For this review, take the finished solid that the model builds, in its own axes (mm). A direction names the side the tool comes from. Give positions to 0.01 mm unless a question says otherwise; leave off trailing zeros. Loops run counter-clockwise (first coordinate to the right, second up) from the corner with the lowest first, then second, coordinate; pieces in that order, holes last. Notation, with made-up numbers: (-10, 34.5) -> (17, 34.5) arc R30 cw to (17, 62.5) -> close; hole circle Ø6 at (-5, 62.5). An arc over 180 degrees is marked (long way). One line per question, with ' | ' between items. Start each with the question number.
(1) Insertion check: P1, Ø4, axis at y = 8, z = -6, coming from the -X side; P2, Ø6, axis at x = -14.5, y = 10.5, coming from the +Z side; P3, Ø6, axis at x = 6.5, y = 6.5, coming from the +Z side. Each pin has a flat end and moves straight along its axis. Give the tip position at first contact, or say it passes through.
(2) Consider section A-A (z = -16). Write out the cut boundary in (x, y), and give its area (3 significant figures).
(3) Consider section B-B (x = -5.5). Write out the cut boundary in (y, z), and give its area (3 significant figures).
(4) Consider section D-D (x = 11). Write out the cut boundary in (y, z).
(5) Wall thickness on probe 1 along Z at (x, y) = (8, 13); probe 2 along Y at (x, z) = (-15, 7); probe 3 along X at (y, z) = (16, -12.5): over which ranges is each line inside the solid? List them lowest first.
(6) Consider section C-C (y = 3). Write out the cut boundary in (x, z).
(7) Tool access review of faces 1 (the flat face through (11, 14, -11)), 2 (the flat face through (-15, 14, 0)), 3 (the cylindrical face through (3.878, 14.465, -9.218)): name each direction out of +Z, -Z, +X, -X, +Y, -Y from which nothing blocks a thin tool from reaching the whole face with its end or side.
(8) Draft analysis for pull direction Z (two halves, no side actions). For faces 4 (the flat face through (0, 0, 0)), 5 (the cylindrical face through (-9.218, 14.465, -3.878)), 6 (the flat face through (-11, 14, -11)), state which applies: +Z half, -Z half, draft (parallel to the pull), parting line (faces both ways), or undercut.
from build123d import *

# Parameters (mm, degrees)
SKETCH1_R                      = 20
EXTRUDE_MECHANISM_PART_1_DEPTH = 17
CUT_START                      = -5
CUT_MECHANISM_PART_1_DEPTH     = 5


with BuildPart() as part:
    # Sketch1 → Extrude (Mechanism Part 1) (new body)
    with BuildSketch(Plane(origin=(0, 0, 0), x_dir=(1, 0, 0), z_dir=(0, 1, 0))):
        with Locations(Location((0, 0, 0), (0, 0, 270))):
            Circle(SKETCH1_R)
    extrude(amount=EXTRUDE_MECHANISM_PART_1_DEPTH)

    # Sketch2 → Cut (Mechanism Part 1) (cut)
    with BuildSketch(Plane(origin=(0, 17, 0), x_dir=(1, 0, 0), z_dir=(0, 1, 0)).offset(CUT_START)):
        with BuildLine():
            Line((0, 10), (0, 20))
            ThreePointArc((0, 20), (-7.653668647, 18.47759065), (-14.142135624, 14.142135624))
            Line((-14.142135624, 14.142135624), (-7.071067812, 7.071067812))
            ThreePointArc((-7.071067812, 7.071067812), (-3.826834324, 9.238795325), (0, 10))
        make_face()
        with BuildLine():
            ThreePointArc((20, 0), (18.47759065, 7.653668647), (14.142135624, 14.142135624))
            Line((14.142135624, 14.142135624), (7.071067812, 7.071067812))
            ThreePointArc((7.071067812, 7.071067812), (9.238795325, 3.826834324), (10, 0))
            Line((10, 0), (20, 0))
        make_face()
        with BuildLine():
            ThreePointArc((7.071067812, -7.071067812), (3.826834324, -9.238795325), (0, -10))
            Line((0, -10), (0, -20))
            ThreePointArc((0, -20), (7.653668647, -18.47759065), (14.142135624, -14.142135624))
            Line((14.142135624, -14.142135624), (7.071067812, -7.071067812))
        make_face()
        with BuildLine():
            Line((-10, 0), (-20, 0))
            ThreePointArc((-20, 0), (-18.47759065, -7.653668647), (-14.142135624, -14.142135624))
            Line((-14.142135624, -14.142135624), (-7.071067812, -7.071067812))
            ThreePointArc((-7.071067812, -7.071067812), (-9.238795325, -3.826834324), (-10, 0))
        make_face()
        with BuildLine():
            Line((-7.071067812, -7.071067812), (0, 0))
            Line((0, 0), (-10, 0))
            ThreePointArc((-10, 0), (-9.238795325, -3.826834324), (-7.071067812, -7.071067812))
        make_face()
        with BuildLine():
            Line((-10, 0), (0, 0))
            Line((0, 0), (-7.071067812, 7.071067812))
            ThreePointArc((-7.071067812, 7.071067812), (-9.238795325, 3.826834324), (-10, 0))
        make_face()
        with BuildLine():
            Line((0, 0), (0, 10))
            ThreePointArc((0, 10), (-3.826834324, 9.238795325), (-7.071067812, 7.071067812))
            Line((-7.071067812, 7.071067812), (0, 0))
        make_face()
        with BuildLine():
            ThreePointArc((7.071067812, 7.071067812), (3.826834324, 9.238795325), (0, 10))
            Line((0, 10), (0, 0))
            Line((0, 0), (7.071067812, 7.071067812))
        make_face()
        with BuildLine():
            Line((7.071067812, 7.071067812), (0, 0))
            Line((0, 0), (10, 0))
            ThreePointArc((10, 0), (9.238795325, 3.826834324), (7.071067812, 7.071067812))
        make_face()
        with BuildLine():
            Line((10, 0), (0, 0))
            Line((0, 0), (7.071067812, -7.071067812))
            ThreePointArc((7.071067812, -7.071067812), (9.238795325, -3.826834324), (10, 0))
        make_face()
        with BuildLine():
            Line((7.071067812, -7.071067812), (0, 0))
            Line((0, 0), (0, -10))
            ThreePointArc((0, -10), (3.826834324, -9.238795325), (7.071067812, -7.071067812))
        make_face()
        with BuildLine():
            Line((0, -10), (0, 0))
            Line((0, 0), (-7.071067812, -7.071067812))
            ThreePointArc((-7.071067812, -7.071067812), (-3.826834324, -9.238795325), (0, -10))
        make_face()
    extrude(amount=CUT_MECHANISM_PART_1_DEPTH, mode=Mode.SUBTRACT)


solid = part.part
A:
1) P1: stops at x = -19.6 | P2: stops at z = 16.36 | P3: stops at z = 19.69
2) outline: (-12, 0) -> (12, 0) -> (12, 17) -> (0, 17) -> (0, 12) -> (-12, 12) -> close | area: 348 mm^2
3) outline: (0, -19.23) -> (12, -19.23) -> (12, 8.35) -> (17, 8.35) -> (17, 19.23) -> (0, 19.23) -> close | area: 516 mm^2
4) outline: (0, -16.7) -> (17, -16.7) -> (17, -11) -> (12, -11) -> (12, 0) -> (17, 0) -> (17, 11) -> (12, 11) -> (12, 16.7) -> (0, 16.7) -> close
5) probe 1: z = -18.33 to -8, 6 to 8 | probe 2: y = 0 to 12 | probe 3: x = -15.61 to -12.5, 0 to 12.5
6) outline: circle Ø40 at (0, 0)
7) face 1: +X, +Y | face 2: -X, +Y | face 3: +Z, +Y
8) face 4: draft | face 5: undercut | face 6: -Z half
